Part model, mm, in its own coordinate system. A direction names the side the tool comes from. Coordinates: 2 decimals unless noted, no trailing zeros. Loops run counter-clockwise (first coordinate to the right, second up) from the corner with the lowest first, then second, coordinate; pieces in that order, holes last. Notation, with made-up numbers: M 17.5,45.25 L 63.5,45.25 A32 ccw 63.5,79.25 Z; hole C 58.25,-25 d7. An arc over 180 degrees is marked long. Answer as a JSON object with one key per item and string values. Group by question number.
1. Saw through at A-A on y = 9. Write the cut outline in (x, z) (3 decimals), then the cut area to 3 significant figures.
2. Drop flat-ended pins along their axis: pin 1 Ø4 at (y, z) = (8, -6.5) entering from +X; pin 2 Ø1 at (x, z) = (-33, -9) entering from +Y; pin 3 Ø0.6 at (x, z) = (-33, -7.5) entering from -Y; pin 4 Ø8 at (x, z) = (11.5, -7) entering from +Y. Give the stop position or say it passes through.
3. 3-axis set-ups, long thin cutter, end or side, ignore diameter. For faces 1 (the face through (-23.453, 9, -1)), 2 (the face through (-33, 5.33, -8)), 3 (the face through (-32.343, 9, -8)): which of +Z, -Z, +X, -X, +Y, -Y reach the whole face in a straight line?
4. Saw through at D-D on z = -6.5. Write the cut outline in (x, y), then the cut area to 3 significant figures.
5. Saw through at C-C on x = -25. Write the cut outline in (y, z) (3 decimals), then the cut area to 3 significant figures.
6. Drill centre lines: L1, parallel to Z at x = 10, y = 13 (3 decimals); L2, parallel to Z at x = -24.5, y = 13.75 (3 decimals); L3, parallel to X at y = 7.5, z = -4.5. Where is each one in solid material? Low to high.
7. Saw through at B-B on z = 2. Write the cut outline in (x, y), then the cut area to 3 significant figures.
Autodesk Inventor part; units mm, degrees
ref_plane "YZ Plane" through (0, 0, 0) normal (1, 0, 0) x (0, 1, 0)
ref_plane "XZ Plane" through (0, 0, 0) normal (0, 1, 0) x (-1, 0, 0)
ref_plane "XY Plane" through (0, 0, 0) normal (0, 0, 1) x (1, 0, 0)
sketch "Sketch1" plane through (0, 0, 0) normal (0, 0, 1) x (1, 0, 0)
  line L0 (-23.4532, 11.6803) -> (-23.4532, 6.6003)
  line L1 (-23.4532, 6.6003) -> (16.8687, 4.0703)
  arc A0 (16.8687, 4.0703) -> (16.8687, 14.2103) centre (17.1868, 9.1403) ccw
  line L2 (16.8687, 14.2103) -> (-23.4532, 11.6803)
  line L3 (-5.5783, 9.1403) -> (17.1868, 9.1403) construction
  dimension "d0" = 5.08
  dimension "d1" = 40.64
  dimension "d2" = 5.08
extrude "Extrusion1" add sketch "Sketch1" along normal blind 3.175
sketch "Sketch2" plane through (0, 0, 3.175) normal (0, 0, 1) x (1, 0, 0)
  line L0 (-23.4532, 6.6003) -> (-23.4532, 11.6803)
  arc A0 (16.8687, 4.0703) -> (16.8687, 14.2103) centre (17.1868, 9.1403) ccw
  line L1 (-23.4532, 4.0603) -> (-33.6132, 4.0603)
  line L2 (-33.6132, 4.0603) -> (-33.6132, 14.2203)
  line L3 (-33.6132, 14.2203) -> (-23.4532, 14.2203)
  line L4 (-23.4532, 14.2203) -> (-23.4532, 4.0603)
  line L5 (17.1868, 9.1403) -> (-29.1497, 9.1403) construction
  dimension "d6" = 10.16
  dimension "d7" = 10.16
  dimension "d8" = 5.08
extrude "Extrusion2" add sketch "Sketch2" against normal blind 6.985
sketch "Sketch3" plane through (0, 0, -3.81) normal (0, 0, -1) x (-1, 0, 0)
  line L0 (33.6132, 14.2203) -> (33.6132, 4.0603)
  line L1 (32.3432, 12.9503) -> (33.6132, 12.9503)
  line L2 (33.6132, 12.9503) -> (33.6132, 5.3303)
  line L3 (33.6132, 5.3303) -> (32.3432, 5.3303)
  line L4 (32.3432, 5.3303) -> (32.3432, 12.9503)
  dimension "d11" = 1.27
  dimension "d12" = 7.62
  dimension "d13" = 1.27
extrude "Extrusion3" add sketch "Sketch3" along normal blind 7.62
fillet "Fillet1" radius 6.35 1 edges at (-33.6132, 9.1403, 3.175)
sketch "Sketch4" plane through (-33.6132, 14.2203, -3.81) normal (0, 1, 0) x (1, 0, 0)
  point P0 (10.16, 0)
  point P1 (5.842, -1.905)
  dimension "d17" = 4.318
  dimension "d18" = 1.905
hole "Hole1" at (-27.7712, 14.2203, -1.905) direction (0, -1, 0) diameter 2.54 end through all
properties part number "handle"
Outcome:
{
 "1": {"outline": "M -33.613,-11.43 L -32.343,-11.43 L -32.343,-3.81 L -23.453,-3.81 L -23.453,0 L 22.265,0 L 22.265,3.175 L -27.263,3.175 A6.35 ccw -33.613,-3.175 Z; hole C -27.771,-1.905 d2.54", "area": "212 mm²"},
 "2": {"pin 1": "stops at x = -32.34", "pin 2": "stops at y = 12.95", "pin 3": "stops at y = 5.33", "pin 4": "passes through"},
 "3": {"face 1": "-Z", "face 2": "-Z, +X, -X, -Y", "face 3": "-Z, +X, +Y, -Y"},
 "4": {"outline": "M -33.61,5.33 L -32.34,5.33 L -32.34,12.95 L -33.61,12.95 Z", "area": "9.68 mm²"},
 "5": {"outline": "M 4.06,-3.81 L 14.22,-3.81 L 14.22,3.175 L 4.06,3.175 Z", "area": "71.0 mm²"},
 "6": {"L1": "z = 0 to 3.175", "L2": "z = -3.81 to 3.175", "L3": "x = -33.61 to -32.34"},
 "7": {"outline": "M -30.94,4.06 L -23.45,4.06 L -23.45,6.6 L 16.87,4.07 A5.08 ccw long 16.87,14.21 L -23.45,11.68 L -23.45,14.22 L -30.94,14.22 Z", "area": "427 mm²"}
}
